Could you check a few things on this model? Use its own coordinates, in mm. A direction names the side the tool comes from. Give positions to 0.01 mm unless a question says otherwise; leave off trailing zeros. Order: outer loops, then holes, each group sorted by start corner. A loop starts at its lowest first (then second) coordinate and runs counter-clockwise, first axis right, second up. Notation, with made-up numbers: M 30.5,70 L 72.5,70 A14 cw 72.5,82 Z; hole C -38,7 d9. An arc over 180 degrees is marked long. Answer in a Markdown table with one row per item. Add a question column.
Autodesk Fusion 360 part; units mm, degrees
sketch "Szkic1" plane through (0, 0, 0) normal (0, 0, 1) x (1, 0, 0)
  line L0 (-6, -25) -> (-25, -25)
  line L1 (-25, -25) -> (-25, -8.3)
  line L2 (-25, -8.3) -> (-6, -8.3)
  line L3 (-6, -8.3) -> (-6, -25)
  line L4 (-26, -7.3) -> (-5, -7.3)
  line L5 (-5, -7.3) -> (-5, -26)
  line L6 (-5, -26) -> (-26, -26)
  line L7 (-26, -26) -> (-26, -7.3)
  dimension "d1" = 16.7
  dimension "d2" = 19
  dimension "d3" = 1
  dimension "d4" = 1
  dimension "d5" = 1
  dimension "d6" = 1
extrude "Wyciągnięcie proste1" add sketch "Szkic1" along normal blind 10
extrude "Wyciągnięcie proste2" add sketch "Szkic1" against normal blind 1 contours L0 L1 L2 L3 | L4 L5 L6 L7
extrude "Wyciągnięcie proste3" add 1 faces at (-12, -26, 2.6667) along direction (0, -1, 0) blind 46.3
extrude "Wyciągnięcie proste4" add 1 faces at (-12, -72.3, 2.6667) along direction (0, -1, 0) blind 10
sketch "Szkic2" plane through (0, 0, -1) normal (0, 0, -1) x (1, 0, 0)
  line L0 (-26, 82.3) -> (-26, 7.3)
  line L1 (-26, 7.3) -> (-5, 7.3)
  line L2 (-5, 7.3) -> (-5, 82.3)
  line L3 (-5, 82.3) -> (-26, 82.3)
  line L4 (-26, 82.3) -> (-5, 82.3)
  line L5 (-5, 82.3) -> (-5, 72.3)
  line L6 (-5, 72.3) -> (-26, 72.3)
  line L7 (-26, 72.3) -> (-26, 82.3)
  dimension "d15" = 10
extrude "Wyciągnięcie proste5" add sketch "Szkic2" against normal blind 160 contours L0 L2 L3 L4 L5 L6 L7
equation "d11 = 65 mm - 18.7 mm"
1. Suppose I cut it at D-D on y = -58.5. List the corners of the cut face in (x, z) for me.
2. Suppose I cut it at B-B on y = -15. List the corners of the cut face in (x, z) for me.
3. For faces 5 (the flat face through (-16, -7.3, 4)), 6 (the flat face through (-16, -17, 0)), 7 (the flat face through (-15, -54, 10)), which set-ups out of +Z, -Z, +X, -X, +Y, -Y let a thin tool reach every point of the face, with its end or its side?
4. Thinking about a two-plate mould opening in Y: for faces 1 (the flat face through (-25, -17, 5)), 2 (the flat face through (-5, -75, 61)), 3 (the flat face through (-15, -72.3, 83)), 4 (the flat face through (-16, -8.3, 5)), which applies, pulls with the +Y half, pulls with the -Y half, needs draft (parallel to the pull), parting line crosses it, or undercut?
5. Will these pins go through, and if not, where does the flat tip stop? P1, Ø1, axis at x = -12, y = -59.5, coming from the +Z side; P2, Ø6.5, axis at x = -15.5, z = 54, coming from the +Y side.
6. Suppose I cut it at C-C on z = 71.5. List the corners of the cut face in (x, y) for me, plus the area to 3 significant figures.
7. If I drill on line 1 along Y through (x, z) = (-23.75, 9); line 2 along Y through (x, z) = (-16.75, 30); line 3 along Z through (x, y) = (-19, -10.5), over which ranges is the centre line in solid material (lowest first)? Write a range as [from, to].
8. Suppose I cut it at A-A on x = -9.5. List the corners of the cut face in (y, z) for me, plus the area to 3 significant figures.
Findings below:
| question | item | result |
|---|---|---|
| 1 | outline | M -26,-1 L -5,-1 L -5,10 L -26,10 Z |
| 2 | outline | M -26,-1 L -5,-1 L -5,10 L -6,10 L -6,0 L -25,0 L -25,10 L -26,10 Z |
| 3 | face 5 | +Z, -Z, +X, -X, +Y |
| 3 | face 6 | +Z |
| 3 | face 7 | +Z, +X, -X, +Y |
| 4 | face 1 | undercut |
| 4 | face 2 | needs draft |
| 4 | face 3 | pulls with the +Y half |
| 4 | face 4 | undercut |
| 5 | P1 | z = 10 |
| 5 | P2 | y = -72.3 |
| 6 | outline | M -26,-82.3 L -5,-82.3 L -5,-72.3 L -26,-72.3 Z |
| 6 | area | 210 mm2 |
| 7 | line 1 | [-82.3, -25], [-8.3, -7.3] |
| 7 | line 2 | [-82.3, -72.3] |
| 7 | line 3 | [-1, 0] |
| 8 | outline | M -82.3,-1 L -7.3,-1 L -7.3,10 L -8.3,10 L -8.3,0 L -25,0 L -25,10 L -72.3,10 L -72.3,159 L -82.3,159 Z |
| 8 | area | 2,150 mm2 |
